Part print with two shaded views. Sizes in mm from the minimum x, y, z corner. A direction names the side the tool comes from. Coordinates: 2 decimals unless noted, no trailing zeros. Loops run counter-clockwise (first coordinate to the right, second up) from the corner with the lowest first, then second, coordinate; pieces in that order, holes last. Notation, with made-up numbers: (59, -9) -> (63, -9) arc R24 ccw to (63, 4) -> close; hole circle Ø8 at (11.25, 30.25). An arc over 180 degrees is marked (long way). Write each question's results on one line, items separated by ' | '.
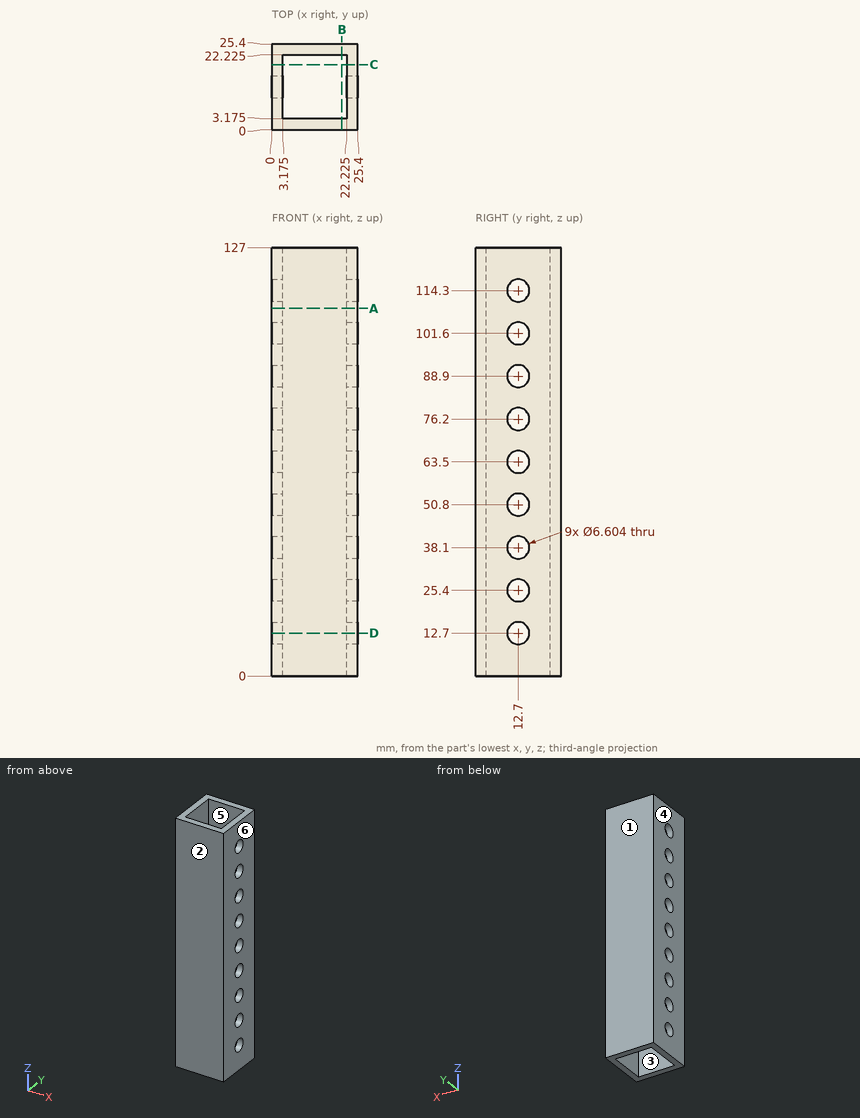
Q1. Pull direction Y, two halves, no side cores. Call the marked faces 1, 2, 3 and 4: +Y half, -Y half, draft (parallel to the pull), parting line (faces both ways), or undercut.
Results are:
face 1: +Y half | face 2: -Y half | face 3: undercut | face 4: draft
Q2. Cut at A-A on z = 109. Write the cut outline in (x, y) (3 decimals).
Results are:
outline: (0, 0) -> (25.4, 0) -> (25.4, 25.4) -> (0, 25.4) -> close; hole (3.175, 3.175) -> (22.225, 3.175) -> (22.225, 22.225) -> (3.175, 22.225) -> close
Q3. Cut at B-B on x = 20.75. Write the cut outline in (y, z) (3 decimals), and give its area (3 significant figures).
Results are:
outline: (0, 0) -> (3.175, 0) -> (3.175, 127) -> (0, 127) -> close; (22.225, 0) -> (25.4, 0) -> (25.4, 127) -> (22.225, 127) -> close | area: 806 mm^2
Q4. Drop a flat-ended pin along its axis: pin 1 (8 mm diameter, centred on x = 5, z = 15.5, fed in from -Y). Give the stop position or say it passes through.
Results are:
pin 1: y = 0
Q5. Cut at D-D on z = 12.7. Write the cut outline in (x, y) (3 decimals).
Results are:
outline: (0, 0) -> (25.4, 0) -> (25.4, 9.398) -> (22.225, 9.398) -> (22.225, 3.175) -> (3.175, 3.175) -> (3.175, 9.398) -> (0, 9.398) -> close; (0, 16.002) -> (3.175, 16.002) -> (3.175, 22.225) -> (22.225, 22.225) -> (22.225, 16.002) -> (25.4, 16.002) -> (25.4, 25.4) -> (0, 25.4) -> close
Q6. Wall check: L1, parallel to Y at x = 18, z = 112 (3 decimals); L2, parallel to Y at x = 2.5, z = 76.2. Give the ranges that are in metal, low to high. Write a range as from..to.
Results are:
L1: 0..3.175, 22.225..25.4 | L2: 0..9.4, 16..25.4
Q7. Which spindle directions (+Z, -Z, +X, -X, +Y, -Y) get a long thin tool onto all of the face, cutting with end or side? Do the marked faces 5 and 6. Say none if no direction does.
Results are:
face 5: +Z, -Z | face 6: +Z, -Z, +X, +Y, -Y
